```python
from build123d import *

# Parameters (mm, degrees)
SKETCH2_W           = 250
SKETCH2_H           = 120
BOSS_EXTRUDE1_DEPTH = 180
SKETCH3_W           = 450
SKETCH3_H           = 180
BOSS_EXTRUDE2_DEPTH = 10
BOSS_EXTRUDE3_DEPTH = 50


with BuildPart() as part:
    # Sketch2 → Boss-Extrude1 (new body)
    with BuildSketch(Plane(origin=(0, 0, 0), x_dir=(1, 0, 0), z_dir=(0, 1, 0))):
        Rectangle(SKETCH2_W, SKETCH2_H)
    extrude(amount=BOSS_EXTRUDE1_DEPTH)

    # Sketch3 → Boss-Extrude2 (add)
    with BuildSketch(Plane(origin=(0, 0, -60), x_dir=(-1, 0, 0), z_dir=(0, 0, -1))):
        with Locations((-100, 90)):
            Rectangle(SKETCH3_W, SKETCH3_H)
    extrude(amount=-BOSS_EXTRUDE2_DEPTH)

    # Sketch4 → Boss-Extrude3 (add)
    with BuildSketch(Plane.XZ):
        with BuildLine():
            Line((125, -50), (300.98, -50))
            Line((300.98, -50), (227.99, 53))
            ThreePointArc((227.99, 53), (212.99, 38), (197.99, 53))
            Line((197.99, 53), (125, -50))
        make_face()
    extrude(amount=-BOSS_EXTRUDE3_DEPTH)


solid = part.part
```
Source: CAD feature listing. Evaluate the final solid. Frame: model axes, mm. A direction names the side the tool comes from. Round coordinates to 2 decimals unless told otherwise and drop trailing zeros. Loops run counter-clockwise (first coordinate to the right, second up) from the corner with the lowest first, then second, coordinate; pieces in that order, holes last. Notation, with made-up numbers: M 39,-34 L 43,-34 A34 ccw 43,-1 Z; hole C -19,49 d9. An arc over 180 degrees is marked long. Put each result on its own line as item: value.
(1) Section C-C, the plane x = 212.99. Return loops of the section in (y, z).
Solutions:
outline: M 0,-60 L 180,-60 L 180,-50 L 50,-50 L 50,38 L 0,38 Z
(2) Section D-D, the plane z = -22. Return loops of the section in (x, y), and give its area (3 significant figures).
Solutions:
outline: M -125,0 L 125,0 L 125,180 L -125,180 Z; M 144.84,0 L 281.14,0 L 281.14,50 L 144.84,50 Z
area: 51,800 mm²
(3) First-contact query: pin 1 (12 mm diameter, centred on x = 191.5, z = 6.5, fed in from +Y); pin 2 (12 mm diameter, centred on y = 143, z = 29.5, fed in from +X); pin 3 (12 mm diameter, centred on y = 37, z = -27, fed in from +X). Flat tips, straight axial feed; report the tip coordinate or a pass-through.
Solutions:
pin 1: y = 50
pin 2: x = 125
pin 3: x = 288.93
(4) Section A-A, the plane z = 16. Return loops of the section in (x, y).
Solutions:
outline: M -125,0 L 125,0 L 125,180 L -125,180 Z; M 171.77,0 L 254.21,0 L 254.21,50 L 171.77,50 Z
(5) Pull-direction query (X, two-part tool) for faces 1 (the face through (125, 89, 6)), 2 (the face through (325, 89, -55)), 3 (the face through (212, 50, -9)); classes: released by +X, released by -X, zero draft, split by the parting line, or undercut.
Solutions:
face 1: undercut
face 2: released by +X
face 3: zero draft
(6) Access query for faces 4 (the face through (162.006, 24.65, 2.221)), 5 (the face through (47, 0, 1)), 6 (the face through (226, 111, -50)). Directions: +Z, -Z, +X, -X, +Y, -Y. A direction counts if a zero-diameter tool reaches every point of the face in a straight line with its end or side. Return the directions, or none.
Solutions:
face 4: +Z, +Y, -Y
face 5: +Z, -Z, +X, -X, -Y
face 6: +Z, +X, +Y
(7) Section B-B, the plane y = 44. Return loops of the section in (x, z), and give its area (3 significant figures).
Solutions:
outline: M -125,-60 L 325,-60 L 325,-50 L 300.98,-50 L 227.99,53 A15 cw 197.99,53 L 125,-50 L 125,60 L -125,60 Z
area: 42,300 mm²
(8) Ray query, line 1 (X direction, y = 170, z = -13.5); line 2 (Z direction, x = 222.5, y = 70); line 3 (Y direction, x = 192, z = -3). Return the intervals inside material, ascending. Write a range as [from, to].
Solutions:
line 1: [-125, 125]
line 2: [-60, -50]
line 3: [0, 50]
